Can you work these out from the model? Positions are in its coordinate system, mm. A direction names the side the tool comes from. Round coordinates to 2 decimals unless told otherwise and drop trailing zeros. Write each loop counter-clockwise with the first axis right and the second up, starting at its lowest first coordinate (ties: lowest second). Pieces come first, ordered by that corner, then holes. Notation, with made-up numbers: M 24,-27.75 L 83,-27.75 A14 ccw 83,-10.75 Z; hole C 10.25,83 d3. An arc over 180 degrees is marked long. Answer in a Markdown table with one row per item. Add a question column.
(1) Suppose I cut it at A-A, the plane z = 0. Write out the boundary of the cut face in (x, y).
(2) I'm going to push flat-ended pins straight in: pin 1 (1.3 mm diameter, centred on x = 57, z = 7.5, fed in from -Y); pin 2 (5 mm diameter, centred on x = 35.5, z = -5, fed in from -Y); pin 3 (4 mm diameter, centred on x = 63.5, y = 5.5, fed in from +Z). Where does each tip first touch, or does it pass through?
(3) For faces 4 (the face through (56, 2.5, 7)), 5 (the face through (58.6, 0, 7.6)), 6 (the face through (56, -2.5, 7)), which set-ups out of +Z, -Z, +X, -X, +Y, -Y let a thin tool reach every point of the face, with its end or its side?
(4) If we mould it in two halves opening along Z, with no side actions, what happens to faces 1 (the face through (31.772, 0, 0)), 2 (the face through (52.972, 0, 8)), 3 (the face through (26.294, -1.822, 5.785))? For each: released by +Z, released by -Z, zero draft, split by the parting line, or undercut.
(5) Suppose I cut it at B-B, the plane x = 45.5. Write out the boundary of the cut face in (y, z).
(6) Suppose I cut it at C-C, the plane x = 26.5. Write out the boundary of the cut face in (y, z), then the cut area to 3 significant figures.
(7) If I drill on probe 1 along X at (y, z) = (1.5, 1.25); probe 2 along Z at (x, y) = (24, 0); probe 3 along Z at (x, y) = (25, 0), over which ranges is the centre line in solid material (lowest first)?
from build123d import *

# Parameters (mm, degrees)
F4_DEPTH = 12.5
F5_R     = 1
F6_DEPTH = 2.5
F7_SIZE  = 0.8
F8_R     = 9.2444577991
F8_R_2   = 8.9
F9_DEPTH = 17.801
F10_R    = 0.5


with BuildPart() as f2:
    # F1 (on Front) → F2 (revolve)
    with BuildSketch(Plane.XZ):
        Polygon((33.6140350877, 6.9), (21.7719298246, 5.55), (21.7719298246, 4.05), (31.7719298246, 4.05), (31.7719298246, 0), (70.7719298246, 0), (70.7719298246, 6.9), align=None)
    revolve(axis=Axis((6, 0, 0), (1, 0, 0)))

    # F3 (on Front) → F4 (cut, symmetric)
    with BuildSketch(Plane.XZ):
        with BuildLine():
            Line((52.9719298246, 6.9), (52.9719298246, 6.2559245818))
            ThreePointArc((52.9719298246, 6.2559245818), (56.7154053617, 5.909998764), (60.4719298246, 6.0576393039))
            Line((60.4719298246, 6.0576393039), (60.4719298246, 6.4))
            Line((60.4719298246, 6.4), (59.6919298246, 6.9))
            Line((59.6919298246, 6.9), (52.9719298246, 6.9))
        make_face()
        with BuildLine():
            Line((60.4719298246, 6.4), (60.4719298246, 6.0576393039))
            ThreePointArc((60.4719298246, 6.0576393039), (62.7387972888, 6.3887114723), (64.9719298246, 6.9))
            Line((64.9719298246, 6.9), (59.6919298246, 6.9))
            Line((59.6919298246, 6.9), (60.4719298246, 6.4))
        make_face()
        with BuildLine():
            ThreePointArc((49.9719298246, 6.9), (51.4632936826, 6.5377365269), (52.9719298246, 6.2559245818))
            Line((52.9719298246, 6.2559245818), (52.9719298246, 6.9))
            Line((52.9719298246, 6.9), (49.9719298246, 6.9))
        make_face()
    extrude(amount=F4_DEPTH, both=True, mode=Mode.SUBTRACT)

    # F5
    f5_edges = [f2.edges().sort_by_distance(p)[0] for p in [
        (57.47193, -3.577709, 5.9),
        (57.47193, 3.577709, 5.9),
    ]]
    fillet(f5_edges, radius=F5_R)

    # F3 (on Front) → F6 (join, symmetric)
    with BuildSketch(Plane.XZ):
        Polygon((52.9719298246, 8.9), (52.9719298246, 6.9), (59.6919298246, 6.9), (56.5719298246, 8.9), align=None)
        with BuildLine():
            Line((52.9719298246, 6.9), (52.9719298246, 6.2559245818))
            ThreePointArc((52.9719298246, 6.2559245818), (56.7154053617, 5.909998764), (60.4719298246, 6.0576393039))
            Line((60.4719298246, 6.0576393039), (60.4719298246, 6.4))
            Line((60.4719298246, 6.4), (59.6919298246, 6.9))
            Line((59.6919298246, 6.9), (52.9719298246, 6.9))
        make_face()
        with BuildLine():
            Line((52.9719298246, 6.2559245818), (52.9719298246, 4.9))
            Line((52.9719298246, 4.9), (60.4719298246, 4.9))
            Line((60.4719298246, 4.9), (60.4719298246, 6.0576393039))
            ThreePointArc((60.4719298246, 6.0576393039), (56.7154053617, 5.909998764), (52.9719298246, 6.2559245818))
        make_face()
    extrude(amount=F6_DEPTH, both=True)

    # F7
    f7_edges = [f2.edges().sort_by_distance(p)[0] for p in [
        (70.77193, 0, -6.9),
    ]]
    chamfer(f7_edges, length=F7_SIZE)

    # F8 (on face) → F9 (cut, through all)
    with BuildSketch(Plane(origin=(52.9719298246, 0, 0), x_dir=(0, -1, 0), z_dir=(-1, 0, 0))):
        Circle(F8_R)
        Circle(F8_R_2, mode=Mode.SUBTRACT)
    extrude(amount=-F9_DEPTH, mode=Mode.SUBTRACT)

    # F10
    f10_edges = [f2.edges().sort_by_distance(p)[0] for p in [
        (56.718854, -1.291345, 8.805818),
        (56.718854, 1.291345, 8.805818),
    ]]
    fillet(f10_edges, radius=F10_R)


solid = f2.part
Calculated:
| question | item | result |
|---|---|---|
| 1 | outline | M 21.77,-5.55 L 33.61,-6.9 L 69.97,-6.9 L 70.77,-6.1 L 70.77,6.1 L 69.97,6.9 L 33.61,6.9 L 21.77,5.55 L 21.77,4.05 L 31.77,4.05 L 31.77,-4.05 L 21.77,-4.05 Z |
| 2 | pin 1 | y = -2.5 |
| 2 | pin 2 | y = -6.43 |
| 2 | pin 3 | z = 5.95 |
| 3 | face 4 | +Z, +Y |
| 3 | face 5 | +Z, +Y, -Y |
| 3 | face 6 | +Z, -Y |
| 4 | face 1 | undercut |
| 4 | face 2 | zero draft |
| 4 | face 3 | split by the parting line |
| 5 | outline | C 0,0 d13.8 |
| 6 | outline | C 0,0 d12.18; hole C 0,0 d8.1 |
| 6 | area | 64.9 mm² |
| 7 | probe 1 | 31.77 to 70.77 |
| 7 | probe 2 | -5.8 to -4.05, 4.05 to 5.8 |
| 7 | probe 3 | -5.92 to -4.05, 4.05 to 5.92 |
